Input: part model. Units: mm. Frame: model coordinates. Face numbers are marked on the shaded views. A direction names the side the tool comes from. Give positions to 0.01 mm unless a question says otherwise; leave off trailing zeros. Write each loop counter-clockwise with the first axis right and the second up, starting at its lowest first coordinate (ties: lowest second). Pieces come first, ordered by that corner, then holes. Notation, with made-up numbers: (33.25, -10.75) -> (51.25, -10.75) arc R17 ccw to (51.25, 16.25) -> close; hole circle Ø10 at (1.5, 68). An arc over 180 degrees is marked (long way). Answer as a JSON object with one key per item and string values. Group by question number.
Autodesk Inventor part; units mm, degrees
ref_plane "YZ Plane" through (0, 0, 0) normal (1, 0, 0) x (0, 1, 0)
ref_plane "XZ Plane" through (0, 0, 0) normal (0, 1, 0) x (-1, 0, 0)
ref_plane "XY Plane" through (0, 0, 0) normal (0, 0, 1) x (1, 0, 0)
sketch "Sketch1" plane through (0, 0, 0) normal (0, 1, 0) x (-1, 0, 0)
  line L0 (8, 10) -> (-8, 10)
  line L1 (-10, 8) -> (-10, -8)
  line L2 (-8, -10) -> (8, -10)
  line L3 (10, -8) -> (10, 8)
  line L4 (10, 10) -> (-10, -10) construction
  line L5 (-10, 10) -> (10, -10) construction
  line L6 (8, 8) -> (-8, 8)
  line L7 (-8, 8) -> (-8, -8)
  line L8 (-8, -8) -> (8, -8)
  line L9 (8, -8) -> (8, 8)
  arc A0 (10, 8) -> (8, 10) centre (8, 8) ccw
  arc A1 (8, -10) -> (10, -8) centre (8, -8) ccw
  arc A2 (-10, -8) -> (-8, -10) centre (-8, -8) ccw
  arc A3 (-8, 10) -> (-10, 8) centre (-8, 8) ccw
  point P0 (0, 0)
  dimension "d0" = 20
  dimension "d1" = 20
  dimension "d2" = 2
  dimension "d3" = 2
extrude "Extrusion1" add sketch "Sketch1" along normal blind 152
sketch "Sketch2" plane through (10, 0, 8) normal (1, 0, 0) x (0, 0, -1)
  line L0 (0, 0) -> (0, 152)
  line L1 (16, 0) -> (16, 152)
  line L2 (0, 0) -> (16, 0)
  line L3 (0, 152) -> (16, 152)
  line L4 (8, 29.2747) -> (8, 0) construction
  line L5 (8, 127) -> (8, 177) construction
  line L6 (8, 102) -> (8, 202) construction
  line L7 (8, 77) -> (8, 227) construction
  line L8 (8, 52) -> (8, 252) construction
  point P0 (8, 0)
  point P1 (8, 140)
  point P2 (8, 10)
  point P3 (3, 127)
  point P4 (3, 102)
  point P5 (3, 77)
  point P6 (3, 52)
  point P7 (3, 27)
  point P8 (13, 127)
  point P9 (13, 102)
  point P10 (13, 77)
  point P11 (13, 52)
  point P12 (13, 27)
  point P13 (3, 147)
  point P14 (13, 147)
  point P15 (8, 76)
  dimension "d6" = 140
  dimension "d7" = 8
  dimension "d22" = 142
  dimension "d23" = 5
  dimension "d24" = 127
  dimension "d27" = 127
  dimension "d130" = 10
  dimension "d159" = 147
  dimension "d160" = 76
hole "Hole1" at (10, 140, 0) at (10, 10, 0) direction (-1, 0, 0) diameter 2.45 depth 2
pattern_circular "Circular Pattern1" count 4 over 360 about axis through (0, -10, 0) along (0, 1, 0) of "Hole1"
thread "Thread1"
thread "Thread2"
hole "Hole2" at (10, 27, 5) at (10, 27, -5) at (10, 52, -5) at (10, 52, 5) at (10, 77, -5) at (10, 77, 5) at (10, 102, 5) at (10, 102, -5) at (10, 127, 5) at (10, 127, -5) direction (-1, 0, 0) diameter 2.45 depth 2
thread "Thread3"
thread "Thread4"
thread "Thread5"
thread "Thread6"
thread "Thread7"
thread "Thread8"
thread "Thread9"
thread "Thread10"
thread "Thread11"
thread "Thread12"
thread "Thread13"
pattern_circular "Circular Pattern2" count 4 over 360 about axis through (0, -10, 0) along (0, 1, 0) of "Hole2"
thread "Thread14"
thread "Thread15"
thread "Thread16"
thread "Thread17"
thread "Thread18"
thread "Thread19"
thread "Thread20"
thread "Thread21"
thread "Thread22"
thread "Thread23"
thread "Thread24"
thread "Thread25"
thread "Thread26"
thread "Thread27"
thread "Thread28"
thread "Thread29"
thread "Thread30"
thread "Thread31"
thread "Thread32"
thread "Thread33"
thread "Thread34"
thread "Thread35"
thread "Thread36"
thread "Thread37"
thread "Thread38"
thread "Thread39"
thread "Thread40"
thread "Thread41"
thread "Thread42"
thread "Thread43"
thread "Thread44"
thread "Thread45"
thread "Thread46"
hole "Hole3" at (10, 147, 5) at (10, 147, -5) direction (-1, 0, 0) diameter 2.45 depth 2
thread "Thread47"
thread "Thread48"
pattern_circular "Circular Pattern3" count 4 over 360 about axis through (0, -10, 0) along (0, 1, 0) of "Hole3"
thread "Thread49"
thread "Thread50"
thread "Thread51"
thread "Thread52"
thread "Thread53"
thread "Thread54"
properties part number "verticalaxle"
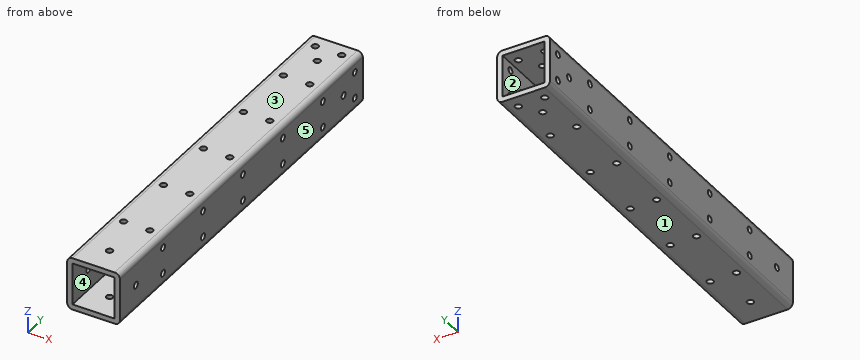
1. Mould query, pull axis X, two halves, no side actions, for the marked faces 3, 4 and 5. Classes: pulls with the +X half, pulls with the -X half, needs draft (parallel to the pull), parting line crosses it, or undercut.
2. Contact query for a flat-ended pin moving along its axis: pin 1 Ø2 at (y, z) = (127, 5) entering from +X. Output: stop coordinate, or through.
3. Reachability of the marked faces 1 and 2 from +Z, -Z, +X, -X, +Y, -Y: full face, straight path, thin tool, end or side. Return the list, or none.
4. Section A-A (y = 93). Return the cut outline in (x, z), plus the area to 3 significant figures.
5. Line query: line 1 (Z direction, x = 4.25, y = 15); line 2 (Y direction, x = 0.25, z = -8.5). Output: solid intervals per line, ascending.
Working result:
{
 "1": {"face 3": "needs draft", "face 4": "undercut", "face 5": "pulls with the +X half"},
 "2": {"pin 1": "passes through"},
 "3": {"face 1": "-Z, +X, -X, +Y, -Y", "face 2": "+Y, -Y"},
 "4": {"outline": "(-10, -8) arc R2 ccw to (-8, -10) -> (8, -10) arc R2 ccw to (10, -8) -> (10, 8) arc R2 ccw to (8, 10) -> (-8, 10) arc R2 ccw to (-10, 8) -> close; hole (-8, -8) -> (8, -8) -> (8, 8) -> (-8, 8) -> close", "area": "141 mm^2"},
 "5": {"line 1": "z = -10 to -8, 8 to 10", "line 2": "y = 0 to 8.8, 11.2 to 138.8, 141.2 to 152"}
}
